Input: dimensioned drawing with shaded views. Units: mm. Origin: part minimum x, y, z. A direction names the side the tool comes from. Give positions to 0.01 mm unless a question says otherwise; leave off trailing zeros. Write each loop counter-clockwise with the first axis right and the second up, starting at its lowest first coordinate (ties: lowest second). Pieces come first, ordered by that corner, then holes. Notation, with made-up numbers: (15.5, 10.5) - (57.5, 10.5) arc R23 cw to (57.5, 34.5) - close; hole circle Ø6 at (-27.75, 76). An arc over 180 degrees is marked (long way). Answer as a JSON object with one key per item and string values. Group by question number.
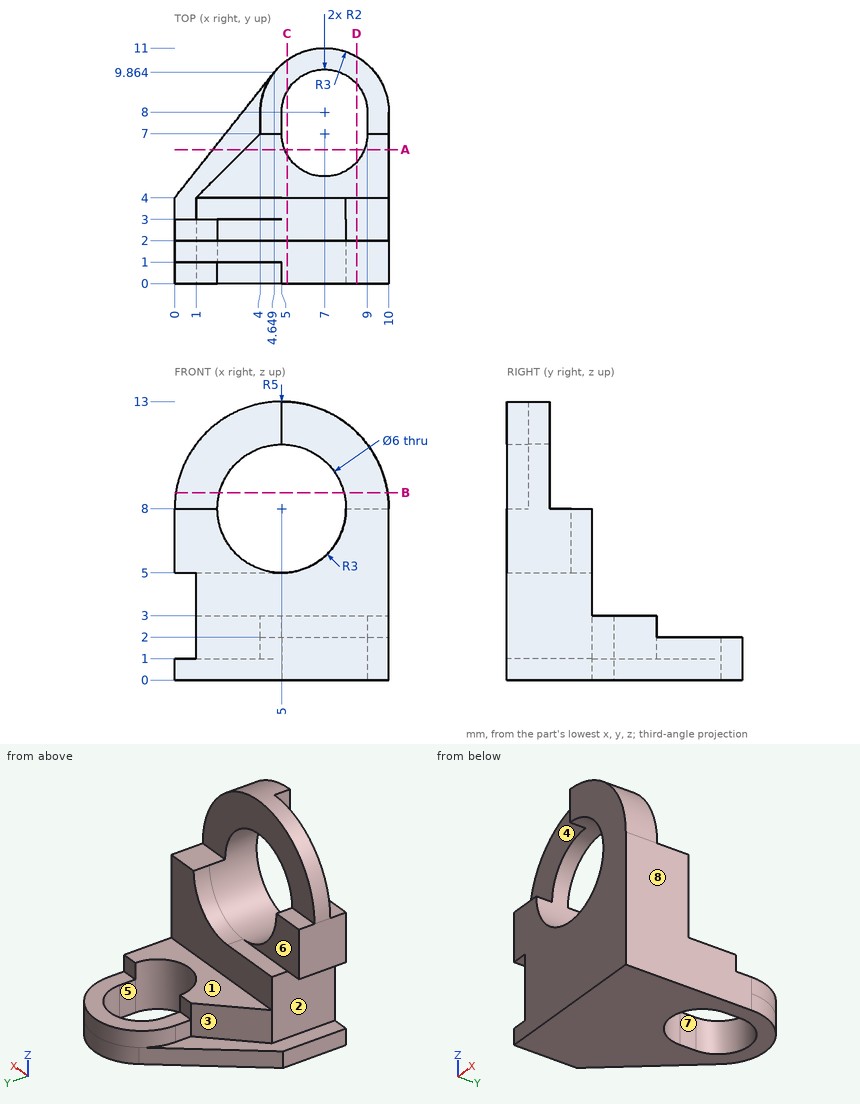
1) Cut plane D-D on x = 8.5. Return the cut outline in (y, z).
2) Reachability of the marked faces 1, 2, 3, 4 and 5 from +Z, -Z, +X, -X, +Y, -Y: full face, straight path, thin tool, end or side. Return the list, or none.
3) Cut plane B-B on z = 8.75. Return the cut outline in (x, y) (1 decimal).
4) Cut plane A-A on y = 6.25. Return the cut outline in (x, z), and give its area (3 significant figures).
5) Line query: line 1 along Z through (x, y) = (5, 1.75); line 2 along X through (y, z) = (1.05, 8); line 3 along Z through (x, y) = (1.25, 0.75). Output: solid intervals per line, ascending. Write a range as from..to.
6) Cut plane C-C on x = 5.25. Return the cut outline in (y, z), and give its area (3 significant figures).
7) Mould query, pull axis Y, two halves, no side actions, for the marked faces 6, 7 and 8. Classes: +Y half, -Y half, draft (parallel to the pull), parting line (faces both ways), or undercut.
8) Pin query (flat end, axial travel): P1, Ø1.6, axis at x = 9.5, y = 3, coming from the +Z side; P2, Ø5.5, axis at x = 7.5, z = 5, coming from the +Y side; P3, Ø2.5, axis at x = 3, z = 6, coming from the +Y side; P4, Ø3, axis at y = 8, z = 6, coming from the -X side. Return the tip coordinate at first contact, or that it passes through.
Filled in:
{
 "1": {"outline": "(0, 0) - (5.68, 0) - (5.68, 3) - (4, 3) - (4, 8) - (2, 8) - (2, 11.57) - (0, 11.57) - close; (9.32, 0) - (10.6, 0) - (10.6, 2) - (9.32, 2) - close"},
 "2": {"face 1": "+Z, +X, -X, +Y", "face 2": "-X, +Y, -Y", "face 3": "+Z, -X, +Y", "face 4": "+Z, -X, -Y", "face 5": "+Z, -Z"},
 "3": {"outline": "(0.1, 1) - (2.1, 1) - (2.1, 2) - (0.1, 2) - close; (7.9, 0) - (9.9, 0) - (9.9, 2) - (7.9, 2) - close"},
 "4": {"outline": "(1.78, 0) - (5.15, 0) - (5.15, 3) - (3.25, 3) - (3.25, 1) - (1.78, 1) - close; (8.85, 0) - (10, 0) - (10, 3) - (8.85, 3) - close", "area": "10.6 mm²"},
 "5": {"line 1": "z = 0..5, 11..13", "line 2": "x = 0..2, 8..10", "line 3": "z = 0..8"},
 "6": {"outline": "(0, 0) - (6.03, 0) - (6.03, 3) - (4, 3) - (4, 5.01) - (0, 5.01) - close; (0, 10.99) - (2, 10.99) - (2, 12.99) - (0, 12.99) - close; (8.97, 0) - (10.44, 0) - (10.44, 2) - (8.97, 2) - close", "area": "33.1 mm²"},
 "7": {"face 6": "+Y half", "face 7": "undercut", "face 8": "draft"},
 "8": {"P1": "stops at z = 8", "P2": "stops at y = 7", "P3": "stops at y = 4", "P4": "passes through"}
}
